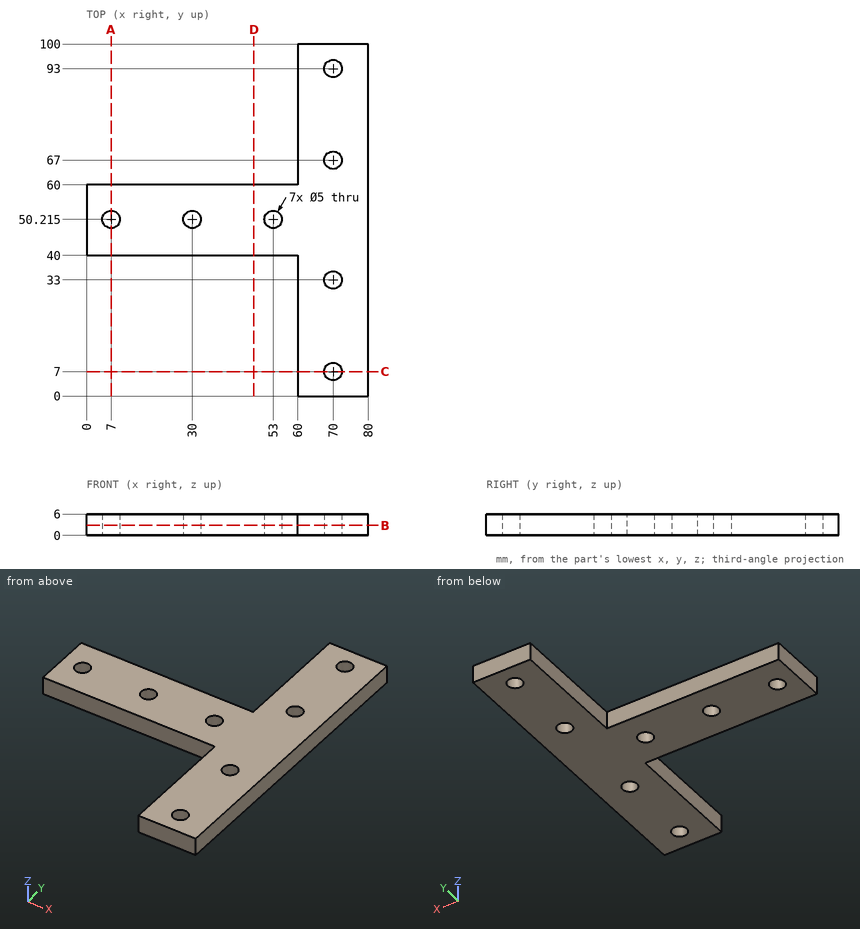
Part print with two shaded views. Sizes in mm from the minimum x, y, z corner. Round coordinates to 2 decimals unless told otherwise and drop trailing zeros. Order: outer loops, then holes, each group sorted by start corner. A loop starts at its lowest first (then second) coordinate and runs counter-clockwise, first axis right, second up. Notation, with made-up numbers: M 26.25,47 L 47.25,47 A34 cw 47.25,85 Z; hole C 77,33 d6. An arc over 180 degrees is marked long. Answer in a Markdown table with one row per item. Add a question column.
Q1. Cut at A-A on x = 7. Give the cut face in (y, z) (1 decimal), and give its area (3 significant figures).
Q2. Wall check: L1, parallel to Y at x = 70, z = 2.95; L2, parallel to X at y = 7, z = 4.05; L3, parallel to Y at x = 7, z = 4 (1 decimal). Give the ranges that are in metal, low to high. Write a range as from..to.
Q3. Pin check, flat tips, straight feed: pin 1 (3 mm diameter, centred on x = 72, y = 38, fed in from -Z); pin 2 (2 mm diameter, centred on y = 18, z = 1.5, fed in from -X); pin 3 (3 mm diameter, centred on x = 7, y = 50.21, fed in from -Z). Stop position of each tip, or through.
Q4. Cut at B-B on z = 2.8. Give the cut face in (x, y) (1 decimal), and give its area (3 significant figures).
Q5. Cut at D-D on x = 47.5. Give the cut face in (y, z).
Q6. Cut at C-C on y = 7. Give the cut face in (x, z), and give its area (3 significant figures).
Established:
| question | item | result |
|---|---|---|
| 1 | outline | M 40,0 L 47.7,0 L 47.7,6 L 40,6 Z; M 52.7,0 L 60,0 L 60,6 L 52.7,6 Z |
| 1 | area | 90.0 mm2 |
| 2 | L1 | y = 0..4.5, 9.5..30.5, 35.5..64.5, 69.5..90.5, 95.5..100 |
| 2 | L2 | x = 60..67.5, 72.5..80 |
| 2 | L3 | y = 40..47.7, 52.7..60 |
| 3 | pin 1 | stops at z = 0 |
| 3 | pin 2 | stops at x = 60 |
| 3 | pin 3 | passes through |
| 4 | outline | M 0,40 L 60,40 L 60,0 L 80,0 L 80,100 L 60,100 L 60,60 L 0,60 Z; hole C 7,50.2 d5; hole C 30,50.2 d5; hole C 53,50.2 d5; hole C 70,7 d5; hole C 70,33 d5; hole C 70,67 d5; hole C 70,93 d5 |
| 4 | area | 3,060 mm2 |
| 5 | outline | M 40,0 L 60,0 L 60,6 L 40,6 Z |
| 6 | outline | M 60,0 L 67.5,0 L 67.5,6 L 60,6 Z; M 72.5,0 L 80,0 L 80,6 L 72.5,6 Z |
| 6 | area | 90.0 mm2 |
